Geometry: see drawing. Coordinates: mm, zero at the bounding-box minimum. A direction names the side the tool comes from. Coordinates: 2 decimals unless noted, no trailing zeros. Order: outer loops, then holes, each group sorted by start corner. A loop starts at its lowest first (then second) coordinate and runs counter-clockwise, first axis right, second up.
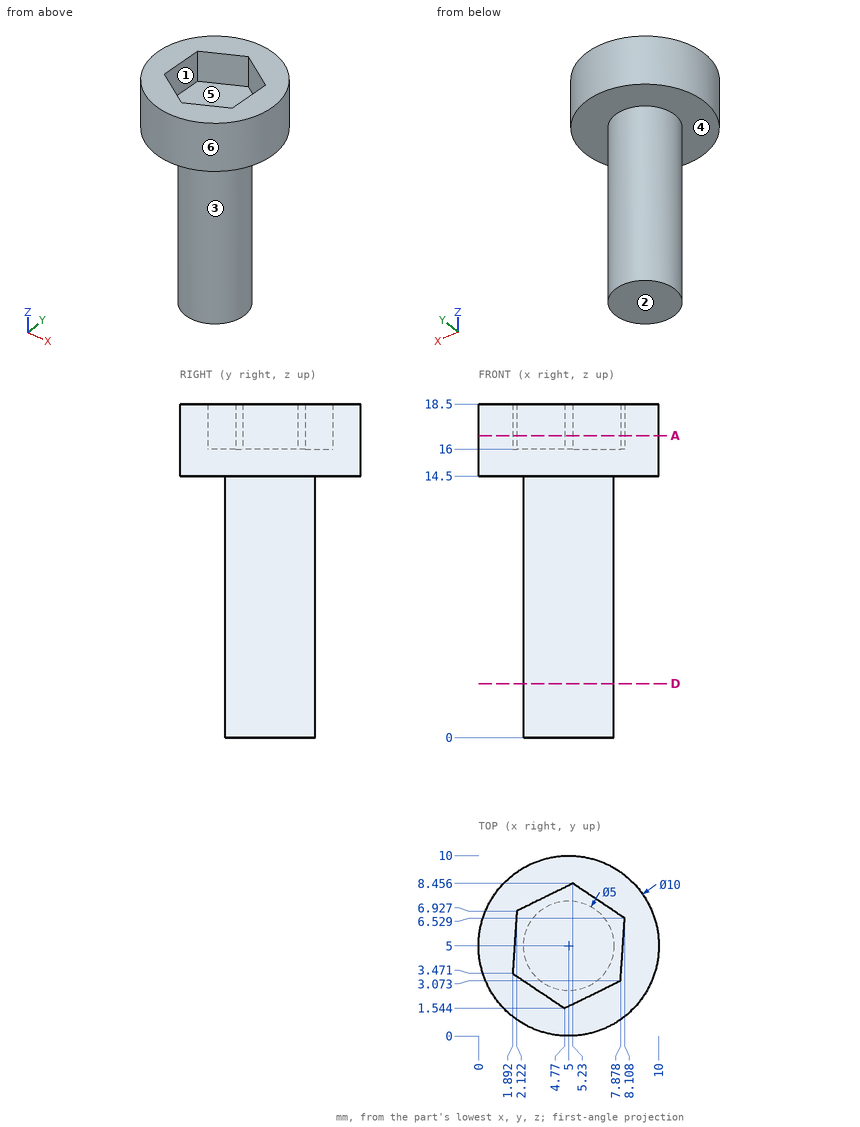
Item 1: Draft query along Y for the marked faces 1, 2 and 3. Return one class per face: pulls with the +Y half, pulls with the -Y half, needs draft (parallel to the pull), parting line crosses it, or undercut.
Response values:
face 1: undercut
face 2: needs draft
face 3: parting line crosses it
Item 2: Pin query (flat end, axial travel): pin 1 Ø2 at (x, z) = (2.5, 13) entering from +Y; pin 2 Ø3 at (x, z) = (7, 15) entering from -Y (1 decimal); pin 3 Ø2 at (x, z) = (5, 2) entering from -Y. Return the tip coordinate at first contact, or that it passes through.
Response values:
pin 1: stops at y = 7
pin 2: stops at y = 0
pin 3: stops at y = 2.5
Item 3: Ray query, probe 1 along Z at (x, y) = (2, 7.25); probe 2 along Y at (x, z) = (3.75, 17) (1 decimal); probe 3 along X at (y, z) = (5, 3). Return the intervals inside material, ascending.
Response values:
probe 1: z = 14.5 to 18.5
probe 2: y = 0.2 to 2.2, 7.7 to 9.8
probe 3: x = 2.5 to 7.5
Item 4: Cut plane A-A on z = 16.75. Return loops of the section in (x, y).
Response values:
outline: circle Ø10 at (5, 5); hole (1.89, 3.47) - (4.77, 1.54) - (7.88, 3.07) - (8.11, 6.53) - (5.23, 8.46) - (2.12, 6.93) - close
Item 5: Cut plane D-D on z = 3. Return loops of the section in (x, y).
Response values:
outline: circle Ø5 at (5, 5)
Item 6: Access query for the marked faces 4, 5 and 6. Directions: +Z, -Z, +X, -X, +Y, -Y. A direction counts if a zero-diameter tool reaches every point of the face in a straight line with its end or side. Return the directions, or none.
Response values:
face 4: -Z
face 5: +Z
face 6: +Z, -Z
